The figure shows three views and two pictorial views of one solid part (mm, origin at its lowest corner). Answer the questions. A direction names the side the tool comes from. Round coordinates to 2 decimals unless told otherwise and drop trailing zeros. One line per item, written item: value.
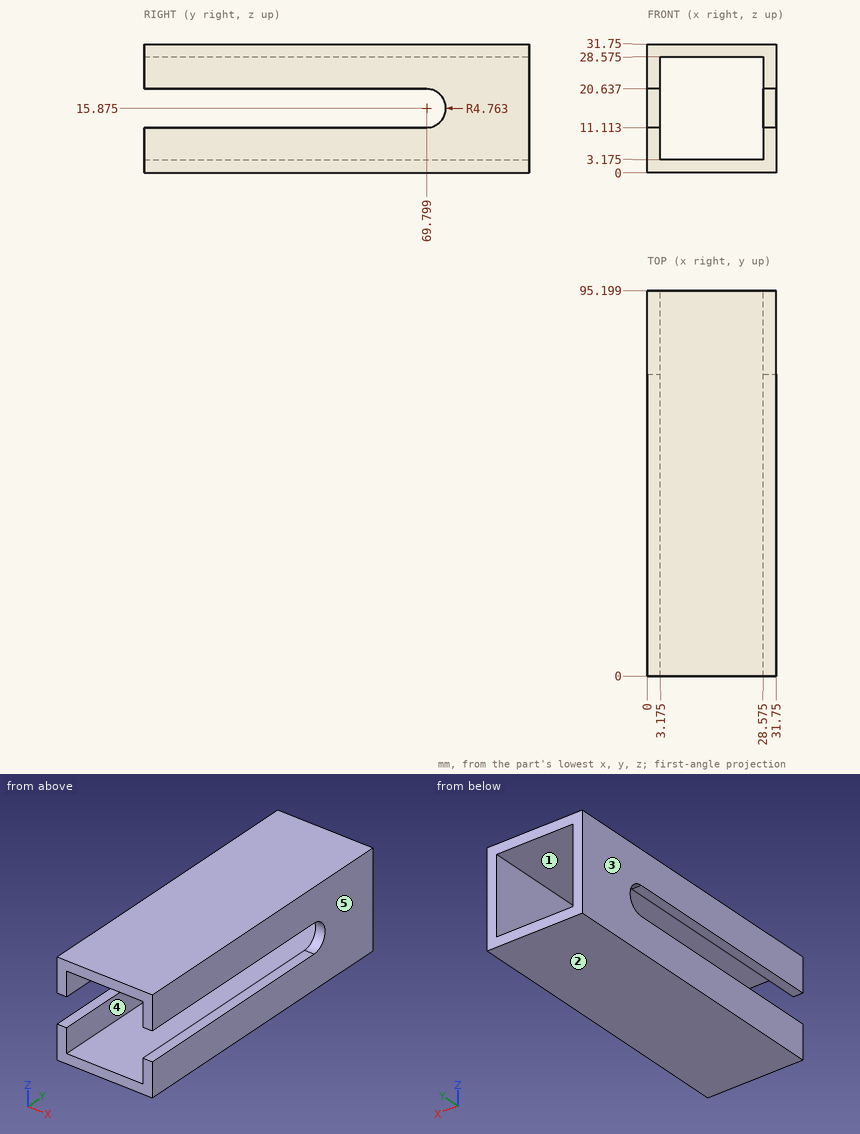
(1) For a pull along X with two mould halves and no side action, classify the marked faces 1, 2 and 3 as pulls with the +X half, pulls with the -X half, needs draft (parallel to the pull), parting line crosses it, or undercut.
Reported:
face 1: undercut
face 2: needs draft
face 3: pulls with the -X half
(2) A tool of negligible diameter and unlimited length cuts with its end or side. For the marked faces 4 and 5, from which of +Z, -Z, +X, -X, +Y, -Y can it reach the whole face along a straight path? Write none if from no direction.
Reported:
face 4: +Y, -Y
face 5: +Z, -Z, +X, +Y, -Y
(3) Flat-ended cylindrical pins translate along their axes: pin 1 Ø7.5 at (y, z) = (40.5, 14.5) entering from -X; pin 2 Ø8 at (x, z) = (24.5, 24) entering from -Y. Find the tip coordinate at first contact, or state that the pin passes through.
Reported:
pin 1: stops at x = 0
pin 2: passes through
(4) Consider probe 1 along Z at (x, y) = (30, 23). Determine where the line is inside the solid, lowest interval first.
Reported:
probe 1: z = 0 to 11.11, 20.64 to 31.75
